Geometry check sheet. Reference: drawing and pictorial views, mm from the part's lowest x, y, z. A direction names the side the tool comes from. Coordinates: 2 decimals unless noted, no trailing zeros. Write each loop counter-clockwise with the first axis right and the second up, starting at its lowest first coordinate (ties: lowest second). Pieces come first, ordered by that corner, then holes. Notation, with made-up numbers: (67, 75) -> (83, 75) arc R31 ccw to (83, 101) -> close; hole circle Ø10 at (1, 15.25). An arc over 180 degrees is marked (long way). Put each result on its own line as item: value.
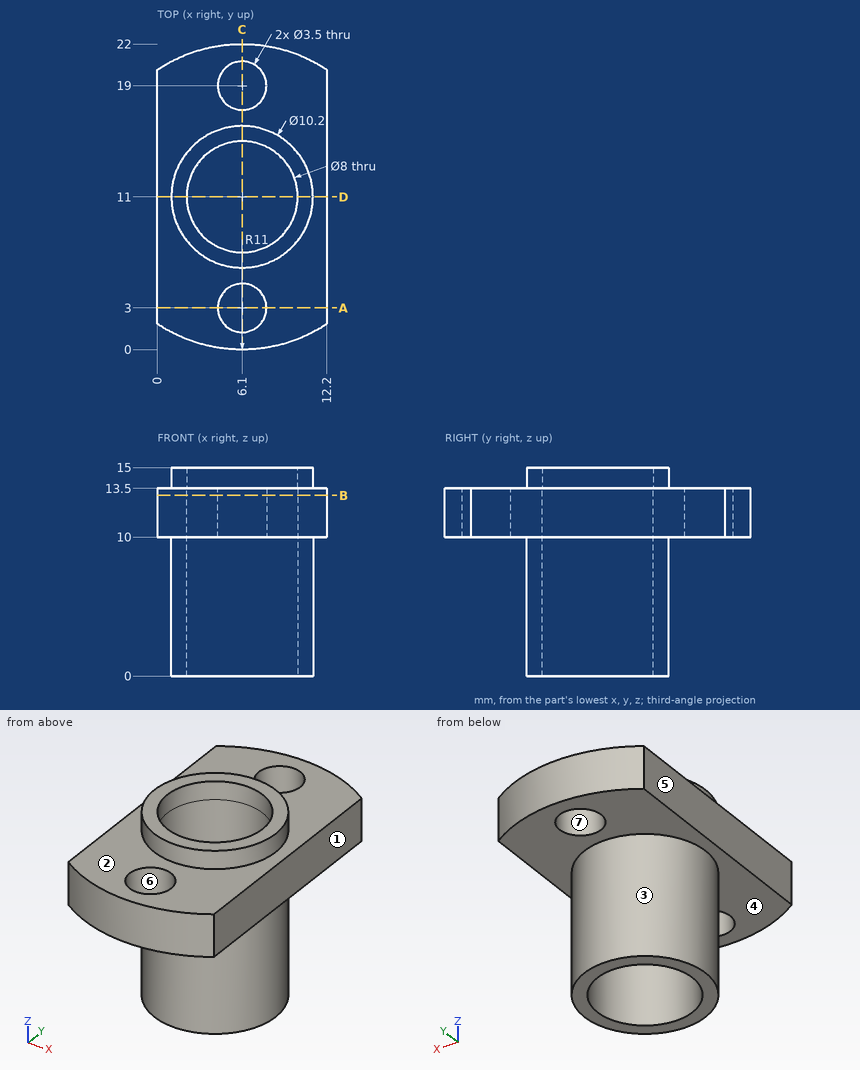
Q1. Tool access check on the marked faces 1, 2 and 3. Record the directions out of +Z, -Z, +X, -X, +Y, -Y that give a thin tool (end or side, any length) a straight path to the whole face; none if there is none.
Recorded:
face 1: +Z, -Z, +X, +Y, -Y
face 2: +Z
face 3: -Z
Q2. Material ranges on line 1 along Y through (x, z) = (7, 11.5); line 2 along Y through (x, z) = (4.5, 11); line 3 along X through (y, z) = (14.5, 1.75), recorded low to high.
Recorded:
line 1: y = 0.04 to 1.5, 4.5 to 7.1, 14.9 to 17.5, 20.5 to 21.96
line 2: y = 0.12 to 2.29, 3.71 to 7.33, 14.67 to 18.29, 19.71 to 21.88
line 3: x = 2.39 to 4.16, 8.04 to 9.81
Q3. Depth check by flat-ended pin: P1, Ø4, axis at y = 5.5, z = 4.5, coming from the +X side; P2, Ø1, axis at x = 4.5, z = 4.5, coming from the -Y side; P3, Ø5, axis at y = 7.5, z = 6.5, coming from the +X side. Enter the tip coordinate at first touch or a pass-through.
Recorded:
P1: stops at x = 9.81
P2: stops at y = 6.02
P3: stops at x = 11.1
Q4. Cross-section at C-C (x = 6.1). Record the cut outline in (y, z), plus the area to 3 significant figures.
Recorded:
outline: (0, 10) -> (1.25, 10) -> (1.25, 13.5) -> (0, 13.5) -> close; (4.75, 10) -> (5.9, 10) -> (5.9, 0) -> (7, 0) -> (7, 15) -> (5.9, 15) -> (5.9, 13.5) -> (4.75, 13.5) -> close; (15, 0) -> (16.1, 0) -> (16.1, 10) -> (17.25, 10) -> (17.25, 13.5) -> (16.1, 13.5) -> (16.1, 15) -> (15, 15) -> close; (20.75, 10) -> (22, 10) -> (22, 13.5) -> (20.75, 13.5) -> close
area: 49.8 mm2
Q5. Cross-section at A-A (y = 3). Record the cut outline in (x, z).
Recorded:
outline: (0, 10) -> (4.35, 10) -> (4.35, 13.5) -> (0, 13.5) -> close; (7.85, 10) -> (12.2, 10) -> (12.2, 13.5) -> (7.85, 13.5) -> close
Q6. Cross-section at B-B (z = 13). Record the cut outline in (x, y).
Recorded:
outline: (0, 1.85) arc R11 ccw to (12.2, 1.85) -> (12.2, 20.15) arc R11 ccw to (0, 20.15) -> close; hole circle Ø8 at (6.1, 11); hole circle Ø3.5 at (6.1, 3); hole circle Ø3.5 at (6.1, 19)
Q7. Cross-section at D-D (y = 11). Record the cut outline in (x, z).
Recorded:
outline: (0, 10) -> (1, 10) -> (1, 0) -> (2.1, 0) -> (2.1, 15) -> (1, 15) -> (1, 13.5) -> (0, 13.5) -> close; (10.1, 0) -> (11.2, 0) -> (11.2, 10) -> (12.2, 10) -> (12.2, 13.5) -> (11.2, 13.5) -> (11.2, 15) -> (10.1, 15) -> close
Q8. Mould release check, pull along X, two halves, no side actions. Record for the marked faces 4, 5, 6 and 7: released by +X, released by -X, zero draft, split by the parting line, or undercut.
Recorded:
face 4: zero draft
face 5: released by -X
face 6: undercut
face 7: undercut
